Can you work these out from the model? Positions are in its coordinate system, mm. A direction names the side the tool comes from. Coordinates: 2 decimals unless noted, no trailing zeros. Loops run counter-clockwise (first coordinate to the right, second up) from the corner with the lowest first, then second, coordinate; pieces in that order, holes last. Notation, with made-up numbers: (64, 51) -> (74, 51) arc R24 cw to (74, 61) -> close; hole circle Ø10 at (61.5, -39.75). An arc over 180 degrees is marked (long way). Use one line per item in the form item = value. Start each with the question number.
(1) Imagine slicing it at A-A (z = 10). List the corners of the cut face in (x, y) for me, plus the area to 4 significant figures.
(2) I'm going to push flat-ended pins straight in: pin 1 (14 mm diameter, centred on x = 10, z = 8.5, fed in from +Y); pin 2 (6.5 mm diameter, centred on x = -17, y = -16.5, fed in from -Z); pin 3 (2 mm diameter, centred on x = -0.5, y = -22.5, fed in from -Z); pin 4 (1 mm diameter, centred on x = -17, y = -41.5, fed in from +Z). Where does each tip first touch, or does it pass through?
(3) On a 3-axis mill with a long thin cutter (end or side, diameter ignored), from which of +Z, -Z, +X, -X, +Y, -Y can I reach the whole of each face in a straight line? I mean faces 5 (the flat face through (-5.589, -27.15, 23.368)), 6 (the flat face through (21, -27, 14.682)), 7 (the flat face through (-8.194, -27.115, 33.646)). Say none if no direction works.
(4) Imagine slicing it at C-C (y = -8.5). List the corners of the cut face in (x, z) for me, plus the area to 3 significant figures.
(5) Imagine slicing it at D-D (z = 26.5). State how many separate pieces and enclosed holes the cut face has, plus the area to 3 significant figures.
(6) I need wall thicknesses on line 1 (Z direction, x = 0, y = -53); line 2 (X direction, y = -49, z = 2); line 3 (Y direction, x = 21.5, z = 29). Which ranges of each line are inside material? Lowest first, please. Write a range as [from, to].
(7) Thinking about a two-plate mould opening in Y: for faces 1 (the flat face through (0, -55, 15)), 2 (the flat face through (0, -27, 30.022)), 3 (the flat face through (0, 0, 15)), 4 (the flat face through (0, -2.5, 8)), which applies, released by +Y, released by -Y, zero draft, split by the parting line, or undercut?
(8) Imagine slicing it at B-B (x = 0). List the corners of the cut face in (y, z) for me.
```python
from build123d import *

# Parameters (mm, degrees)
F1_DEPTH = 55
F2_T     = -2.5
F3_DEPTH = 55
F5_DEPTH = 25
F7_DEPTH = 25
F8_R     = 1.75
F9_DEPTH = 60


with BuildPart() as f1:
    # F0 (on Front) → F1 (new body)
    with BuildSketch(Plane.XZ):
        Polygon((0, 30.0219481358), (0, 0), (25.5, 0), (25.5, 14.6816842611), (15.8114124709, 14.6816842611), (3.4315507477, 30.0219481358), align=None)
        Polygon((-25.5, 0), (0, 0), (0, 30.0219481358), (-3.4315507477, 30.0219481358), (-15.8114124709, 14.6816842611), (-25.5, 14.6816842611), align=None)
    extrude(amount=F1_DEPTH)

    # F2
    f2_openings = [f1.faces().sort_by_distance(p)[0] for p in [
        (0, -27.5, 0),
    ]]
    offset(amount=F2_T, openings=f2_openings, kind=Kind.INTERSECTION)

    # F0 (on Front) → F3 (join)
    with BuildSketch(Plane.XZ):
        Polygon((13.0917496571, 37.3736836002), (3.4315507477, 30.0219481358), (15.8114124709, 14.6816842611), (25.5, 28.9454380277), align=None)
        Polygon((-15.8114124709, 14.6816842611), (-3.4315507477, 30.0219481358), (-13.0917496571, 37.3736836002), (-25.5, 28.9454380277), align=None)
    extrude(amount=F3_DEPTH)

    # F4 (on face) → F5 (cut)
    with BuildSketch(Plane(origin=(21.5044814121, 0, 31.6593752), x_dir=(0.8272166895, 0, -0.5618830382), z_dir=(0.5618830382, 0, 0.8272166895))):
        with BuildLine():
            ThreePointArc((-2.6699250771, -39), (-8.1699250771, -44.5), (-2.6699250771, -50))
            Line((-2.6699250771, -50), (-2.6699250771, -39))
        make_face()
        with BuildLine():
            Line((-2.6699250771, -39), (-2.6699250771, -50))
            ThreePointArc((-2.6699250771, -50), (1.2191622194, -48.3890872965), (2.8300749229, -44.5))
            ThreePointArc((2.8300749229, -44.5), (1.2191622194, -40.6109127035), (-2.6699250771, -39))
        make_face()
        with BuildLine():
            ThreePointArc((-2.6699250771, -25), (-8.1699250771, -30.5), (-2.6699250771, -36))
            Line((-2.6699250771, -36), (-2.6699250771, -25))
        make_face()
        with BuildLine():
            Line((-2.6699250771, -25), (-2.6699250771, -36))
            ThreePointArc((-2.6699250771, -36), (1.2191622194, -34.3890872965), (2.8300749229, -30.5))
            ThreePointArc((2.8300749229, -30.5), (1.2191622194, -26.6109127035), (-2.6699250771, -25))
        make_face()
        with BuildLine():
            Line((-2.6699250771, -22), (-2.6699250771, -11))
            ThreePointArc((-2.6699250771, -11), (-8.1699250771, -16.5), (-2.6699250771, -22))
        make_face()
        with BuildLine():
            ThreePointArc((2.8300749229, -16.5), (1.2191622194, -12.6109127035), (-2.6699250771, -11))
            Line((-2.6699250771, -11), (-2.6699250771, -22))
            ThreePointArc((-2.6699250771, -22), (1.2191622194, -20.3890872965), (2.8300749229, -16.5))
        make_face()
    extrude(amount=-F5_DEPTH, mode=Mode.SUBTRACT)

    # F6 (on face) → F7 (cut)
    with BuildSketch(Plane(origin=(-21.5044814121, 0, 31.6593752), x_dir=(0.8272166895, 0, 0.5618830382), z_dir=(-0.5618830382, 0, 0.8272166895))):
        with BuildLine():
            ThreePointArc((8.1699250771, -10.5), (6.5590123736, -6.6109127035), (2.6699250771, -5))
            Line((2.6699250771, -5), (2.6699250771, -16))
            ThreePointArc((2.6699250771, -16), (6.5590123736, -14.3890872965), (8.1699250771, -10.5))
        make_face()
        with BuildLine():
            Line((2.6699250771, -16), (2.6699250771, -5))
            ThreePointArc((2.6699250771, -5), (-2.8300749229, -10.5), (2.6699250771, -16))
        make_face()
        with BuildLine():
            ThreePointArc((8.1699250771, -24.5), (6.5590123736, -20.6109127035), (2.6699250771, -19))
            Line((2.6699250771, -19), (2.6699250771, -30))
            ThreePointArc((2.6699250771, -30), (6.5590123736, -28.3890872965), (8.1699250771, -24.5))
        make_face()
        with BuildLine():
            Line((2.6699250771, -30), (2.6699250771, -19))
            ThreePointArc((2.6699250771, -19), (-2.8300749229, -24.5), (2.6699250771, -30))
        make_face()
        with BuildLine():
            Line((2.6699250771, -33), (2.6699250771, -44))
            ThreePointArc((2.6699250771, -44), (6.5590123736, -42.3890872965), (8.1699250771, -38.5))
            ThreePointArc((8.1699250771, -38.5), (6.5590123736, -34.6109127035), (2.6699250771, -33))
        make_face()
        with BuildLine():
            ThreePointArc((2.6699250771, -33), (-2.8300749229, -38.5), (2.6699250771, -44))
            Line((2.6699250771, -44), (2.6699250771, -33))
        make_face()
    extrude(amount=-F7_DEPTH, mode=Mode.SUBTRACT)

    # F8 (on face) → F9 (cut)
    with BuildSketch(Plane.XZ.offset(55)):
        with Locations((0, 10)):
            Circle(F8_R)
    extrude(amount=-F9_DEPTH, mode=Mode.SUBTRACT)


solid = f1.part
```
Worked out:
q1.outline = (-25.5, -55) -> (-1.75, -55) -> (-1.75, -52.5) -> (-23, -52.5) -> (-23, -2.5) -> (-1.75, -2.5) -> (-1.75, 0) -> (-25.5, 0) -> close; (1.75, -55) -> (25.5, -55) -> (25.5, 0) -> (1.75, 0) -> (1.75, -2.5) -> (23, -2.5) -> (23, -52.5) -> (1.75, -52.5) -> close
q1.area = 487.5 mm2
q2.pin_1 = 0
q2.pin_2 = 12.18
q2.pin_3 = 27.52
q2.pin_4 = 22.54
q3.face_5 = -Z
q3.face_6 = +X, +Y, -Y
q3.face_7 = +Z, +Y, -Y
q4.outline = (-25.5, 0) -> (-23, 0) -> (-23, 12.18) -> (-14.62, 12.18) -> (-12.78, 14.45) -> (-23.53, 30.28) -> (-25.5, 28.95) -> (-15.81, 14.68) -> (-25.5, 14.68) -> close; (-15.06, 36.04) -> (-6.06, 22.79) -> (-2.24, 27.52) -> (2.24, 27.52) -> (14.62, 12.18) -> (23, 12.18) -> (23, 0) -> (25.5, 0) -> (25.5, 14.68) -> (15.81, 14.68) -> (25.5, 28.95) -> (13.09, 37.37) -> (3.43, 30.02) -> (-3.43, 30.02) -> (-13.09, 37.37) -> close
q4.area = 543 mm2
q5.separate_pieces = 1
q5.enclosed_holes = 7
q5.area = 1,630 mm2
q6.line_1 = [0, 8.25], [11.75, 30.02]
q6.line_2 = [-25.5, -23], [23, 25.5]
q6.line_3 = [-55, -48.1], [-40.9, -34.1], [-26.9, -20.1], [-12.9, 0]
q7.face_1 = released by -Y
q7.face_2 = zero draft
q7.face_3 = released by +Y
q7.face_4 = undercut
q8.outline = (-55, 0) -> (-52.5, 0) -> (-52.5, 8.25) -> (-55, 8.25) -> close; (-55, 11.75) -> (-52.5, 11.75) -> (-52.5, 27.52) -> (-2.5, 27.52) -> (-2.5, 11.75) -> (0, 11.75) -> (0, 30.02) -> (-55, 30.02) -> close; (-2.5, 0) -> (0, 0) -> (0, 8.25) -> (-2.5, 8.25) -> close
